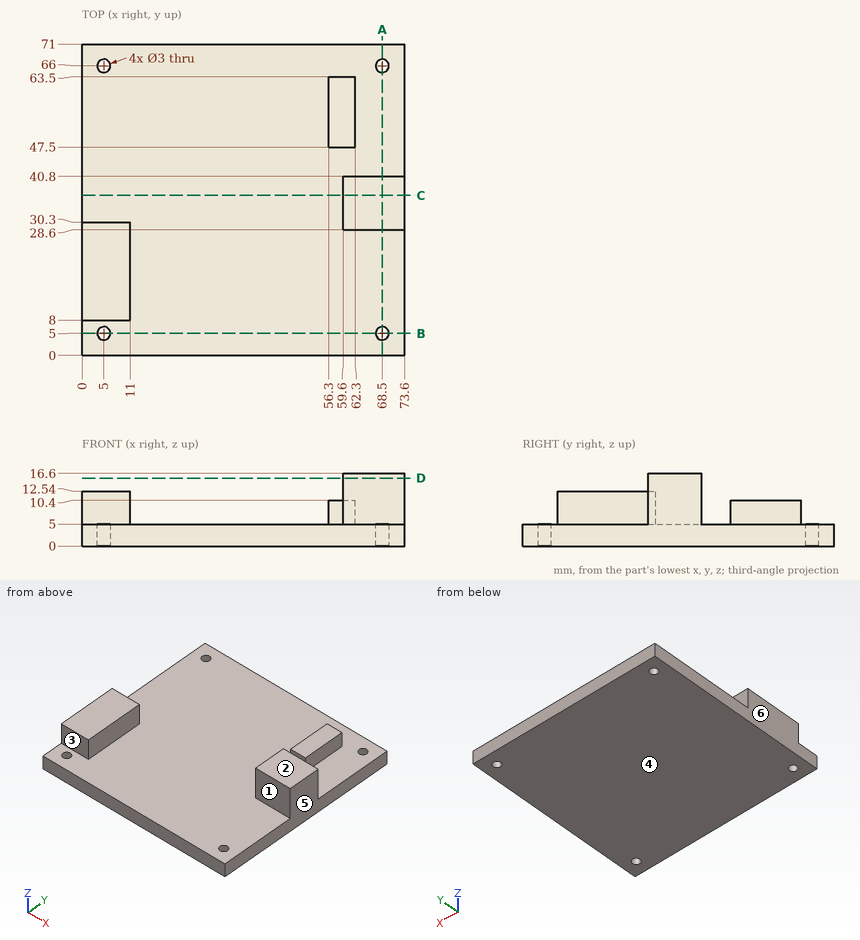
For this review, use the dimensioned drawing (mm, ordinates from the lowest corner) and the shaded views. A direction names the side the tool comes from. Coordinates: 2 decimals unless noted, no trailing zeros. Write each loop counter-clockwise with the first axis right and the second up, starting at its lowest first coordinate (ties: lowest second). Pieces come first, ordered by that corner, then holes. Notation, with made-up numbers: (1.25, 35) - (32.25, 35) arc R32 cw to (32.25, 68) - close; hole circle Ø10 at (-28.75, 87). An arc over 180 degrees is marked (long way). One line per item, written item: value.
1) Add section B-B (y = 5). State the section outline as (x, z) points, plus the area to 3 significant figures.
Answer sheet:
outline: (0, 0) - (3.5, 0) - (3.5, 5) - (0, 5) - close; (6.5, 0) - (67, 0) - (67, 5) - (6.5, 5) - close; (70, 0) - (73.6, 0) - (73.6, 5) - (70, 5) - close
area: 338 mm2
2) Add section D-D (z = 15.5). State the section outline as (x, y) points, plus the area to 3 significant figures.
Answer sheet:
outline: (59.6, 28.6) - (73.6, 28.6) - (73.6, 40.8) - (59.6, 40.8) - close
area: 171 mm2
3) Mouldability with a two-part tool opening along X and no side actions: class the marked faces 4, 5 and 6 as +X half, -X half, draft (parallel to the pull), parting line (faces both ways), or undercut.
Answer sheet:
face 4: draft
face 5: +X half
face 6: -X half
4) Insertion check: pin 1 (1.6 mm diameter, centred on y = 54, z = 7, fed in from +X); pin 2 (2 mm diameter, centred on x = 43, y = 14.5, fed in from -Z); pin 3 (6 mm diameter, centred on y = 16, z = 10, fed in from +X); pin 4 (5 mm diameter, centred on x = 5, y = 66, fed in from +Z). Each pin has a flat end and moves straight along its axis. Give the tip position at first contact, or say it passes through.
Answer sheet:
pin 1: stops at x = 62.3
pin 2: stops at z = 0
pin 3: stops at x = 11
pin 4: stops at z = 5
5) To check wall thickness, follow probe 1 along X at (y, z) = (66, 1.1); probe 2 along Y at (x, z) = (5, 1.05); probe 3 along Z at (x, y) = (44, 47). State the ranges of each line that lie inside material, in increasing order.
Answer sheet:
probe 1: x = 0 to 3.5, 6.5 to 67, 70 to 73.6
probe 2: y = 0 to 3.5, 6.5 to 64.5, 67.5 to 71
probe 3: z = 0 to 5
6) Add section C-C (y = 36.5). State the section outline as (x, z) points.
Answer sheet:
outline: (0, 0) - (73.6, 0) - (73.6, 16.6) - (59.6, 16.6) - (59.6, 5) - (0, 5) - close
7) For the marked faces 1, 2 and 3, list the 3-axis set-ups (+Z, -Z, +X, -X, +Y, -Y) from which the entire face can be reached by the end or side of a thin tool; tool diameter is ignored.
Answer sheet:
face 1: +Z, +X, -Y
face 2: +Z, +X, -X, +Y, -Y
face 3: +Z, +X, -X, -Y
8) Add section A-A (x = 68.5). State the section outline as (y, z) points, plus the area to 3 significant figures.
Answer sheet:
outline: (0, 0) - (3.5, 0) - (3.5, 5) - (0, 5) - close; (6.5, 0) - (64.5, 0) - (64.5, 5) - (40.8, 5) - (40.8, 16.6) - (28.6, 16.6) - (28.6, 5) - (6.5, 5) - close; (67.5, 0) - (71, 0) - (71, 5) - (67.5, 5) - close
area: 467 mm2
